```python
from build123d import *

# Parameters (mm, degrees)
F1_DEPTH = 6


with BuildPart() as f1:
    # F0 (on Front) → F1 (new body)
    with BuildSketch(Plane.XZ):
        Polygon((-136.143627, 115), (-150.429341, 115), (-150.429341, 101.470588), (-144.429341, 101.470588), (-144.429341, 87.941176), (-150.429341, 87.941176), (-150.429341, 74.411765), (-144.429341, 74.411765), (-144.429341, 60.882353), (-150.429341, 60.882353), (-150.429341, 47.352941), (-144.429341, 47.352941), (-144.429341, 33.823529), (-150.429341, 33.823529), (-150.429341, 20.294118), (-144.429341, 20.294118), (-144.429341, 6.764706), (-150.429341, 6.764706), (-150.429341, -6.764706), (-144.429341, -6.764706), (-144.429341, -20.294118), (-150.429341, -20.294118), (-150.429341, -33.823529), (-144.429341, -33.823529), (-144.429341, -47.352941), (-150.429341, -47.352941), (-150.429341, -60.882353), (-144.429341, -60.882353), (-144.429341, -74.411765), (-150.429341, -74.411765), (-150.429341, -87.941176), (-144.429341, -87.941176), (-144.429341, -101.470588), (-150.429341, -101.470588), (-150.429341, -115), (-136.143627, -115), (-136.143627, -109), (-121.857913, -109), (-121.857913, -115), (-107.572198, -115), (-107.572198, -109), (-93.286484, -109), (-93.286484, -115), (-79.00077, -115), (-79.00077, -109), (-64.715055, -109), (-64.715055, -115), (-50.429341, -115), (-50.429341, -109), (-36.143627, -109), (-36.143627, -115), (-21.857913, -115), (-21.857913, -109), (-7.572198, -109), (-7.572198, -115), (6.713516, -115), (6.713516, -109), (20.99923, -109), (20.99923, -115), (35.284945, -115), (35.284945, -109), (49.570659, -109), (49.570659, -115), (63.856373, -115), (63.856373, -109), (78.142087, -109), (78.142087, -115), (92.427802, -115), (92.427802, -109), (106.713516, -109), (106.713516, -115), (120.99923, -115), (120.99923, -109), (135.284945, -109), (135.284945, -115), (149.570659, -115), (149.570659, -101.470588), (143.570659, -101.470588), (143.570659, -87.941176), (149.570659, -87.941176), (149.570659, -74.411765), (143.570659, -74.411765), (143.570659, -60.882353), (149.570659, -60.882353), (149.570659, -47.352941), (144.429341, -47.352941), (144.429341, -33.823529), (150.429341, -33.823529), (150.429341, -20.294118), (144.429341, -20.294118), (144.429341, -6.764706), (150.429341, -6.764706), (150.429341, 6.764706), (144.429341, 6.764706), (144.429341, 20.294118), (150.429341, 20.294118), (150.429341, 33.823529), (144.429341, 33.823529), (144.429341, 47.352941), (150.429341, 47.352941), (150.429341, 60.882353), (144.429341, 60.882353), (144.429341, 74.411765), (149.570659, 74.411765), (149.570659, 87.941176), (143.570659, 87.941176), (143.570659, 101.470588), (149.570659, 101.470588), (149.570659, 115), (135.284945, 115), (135.284945, 109), (120.99923, 109), (120.99923, 115), (106.713516, 115), (106.713516, 109), (92.427802, 109), (92.427802, 115), (78.142087, 115), (78.142087, 109), (63.856373, 109), (63.856373, 115), (49.570659, 115), (49.570659, 109), (35.284945, 109), (35.284945, 115), (20.99923, 115), (20.99923, 109), (6.713516, 109), (6.713516, 115), (-7.572198, 115), (-7.572198, 109), (-21.857913, 109), (-21.857913, 115), (-36.143627, 115), (-36.143627, 109), (-50.429341, 109), (-50.429341, 115), (-64.715055, 115), (-64.715055, 109), (-79.00077, 109), (-79.00077, 115), (-93.286484, 115), (-93.286484, 109), (-107.572198, 109), (-107.572198, 115), (-121.857913, 115), (-121.857913, 109), (-136.143627, 109), align=None)
    extrude(amount=F1_DEPTH)


solid = f1.part
```
Geometry check sheet. Reference: the model listing, model coordinates, mm. A direction names the side the tool comes from. Coordinates: 2 decimals unless noted, no trailing zeros. Write each loop counter-clockwise with the first axis right and the second up, starting at its lowest first coordinate (ties: lowest second). Pieces come first, ordered by that corner, then holes. Notation, with made-up numbers: M 71,82 L 79,82 A17 ccw 79,86 Z; hole C 49.25,-28.5 d11. An arc over 180 degrees is marked long. Use one line per item in the form item = value. Start each with the question number.
1) Set-up check for faces 4 (the flat face through (49.571, -3, -112)), 5 (the flat face through (128, -3, 109)), 6 (the flat face through (-144.429, -3, 41)): record each of +Z, -Z, +X, -X, +Y, -Y from which the full face is reachable in a straight line by a thin tool's end or side.
2) Section check B-B on z = 43. Enter the section's corners in (x, y), and give its area (3 significant figures).
3) Thickness scan on probe 1 along Z at (x, y) = (97.5, -3.8); probe 2 along X at (y, z) = (-2.1, 45.5); probe 3 along X at (y, z) = (-2.1, 98). Record the ranges inside material, lowest first. Write a range as from..to.
4) Release check for a two-part mould opening along X. For faces 1 (the flat face through (147, -3, 6.765)), 2 (the flat face through (-150.429, -3, -27)), 3 (the flat face through (14, -3, -109)) record: pulls with the +X half, pulls with the -X half, needs draft (parallel to the pull), parting line crosses it, or undercut.
5) Section check A-A on z = -91.5. Enter the section's corners in (x, y).
6) Go/stop test with flat-tipped pins: pin 1 Ø3 at (x, y) = (127.5, -3) entering from -Z; pin 2 Ø1.8 at (y, z) = (-2.5, 13) entering from -X; pin 3 Ø2 at (x, y) = (75, -1.5) entering from +Z. Record where each tip stops, or that it passes through.
Responses:
q1.face_4 = -Z, +Y, -Y
q1.face_5 = +Z, +Y, -Y
q1.face_6 = -X, +Y, -Y
q2.outline = M -144.43,-6 L 144.43,-6 L 144.43,0 L -144.43,0 Z
q2.area = 1,730 mm2
q3.probe_1 = -109..109
q3.probe_2 = -144.43..144.43
q3.probe_3 = -144.43..143.57
q4.face_1 = needs draft
q4.face_2 = pulls with the -X half
q4.face_3 = undercut
q5.outline = M -144.43,-6 L 143.57,-6 L 143.57,0 L -144.43,0 Z
q6.pin_1 = -109
q6.pin_2 = -144.43
q6.pin_3 = 109
